Autodesk Inventor part; units mm, degrees
ref_plane "YZ Plane" through (0, 0, 0) normal (1, 0, 0) x (0, 1, 0)
ref_plane "XZ Plane" through (0, 0, 0) normal (0, 1, 0) x (-1, 0, 0)
ref_plane "XY Plane" through (0, 0, 0) normal (0, 0, 1) x (1, 0, 0)
sketch "Sketch1" plane through (0, 0, 0) normal (0, 0, 1) x (1, 0, 0)
  line L0 (-20.32, 1.016) -> (157.7405, 1.016)
  line L1 (-20.32, 1.016) -> (-20.32, 0)
  line L2 (-20.32, 0) -> (174.316, 0)
  line L3 (157.7405, 1.016) -> (158.9661, 1.524)
  line L4 (158.9661, 1.524) -> (174.316, 1.524)
  line L5 (174.316, 1.524) -> (174.316, 0)
  arc A0 (174.316, 1.524) -> (176.856, 4.064) centre (174.316, 4.064) ccw
  line L6 (176.856, 4.064) -> (176.856, 7.009)
  arc A1 (178.38, 7.9375) -> (175.0839, 7.75) centre (177.5921, -7.2764) ccw
  line L7 (176.856, 4.064) -> (179.904, 4.064)
  line L8 (178.38, 4.064) -> (178.38, 7.9375)
  arc A2 (174.316, 0) -> (178.38, 4.064) centre (174.316, 4.064) ccw
  line L9 (175.0839, 7.75) -> (175.0839, 7.3209)
  line L10 (175.0839, 7.3209) -> (176.856, 7.009)
  arc A3 (-19.626, 4.4916) -> (-20.32, 1.016) centre (-11.2701, 1.016) ccw
  line L11 (-19.626, 4.4916) -> (-19.3494, 4.4916)
  line L12 (-19.3494, 4.4916) -> (-18.8257, 3.175)
  line L13 (0, 3.175) -> (4.2213, 3.175)
  line L14 (4.2213, 3.175) -> (5.08, 1.016)
  line L15 (5.08, 1.016) -> (5.08, 0)
  line L16 (0, 3.175) -> (0, 0)
  line L17 (-18.8257, 3.175) -> (0, 3.175)
  line L18 (0, 0) -> (5.08, 0)
  dimension "d1" = 2.032
  dimension "d2" = 3.048
  dimension "d5" = 6.35
  dimension "d11" = 9.0499
  dimension "d12" = 25.4
  dimension "d13" = 5.08
  dimension "d14" = 0.2766
  dimension "d15" = 1.4943
  dimension "d16" = 1.2255
  dimension "d17" = 2.54
  dimension "d18" = 7.9375
  dimension "d19" = 15.2343
  dimension "d20" = 6.5922
  dimension "d21" = 198.7
revolve "Revolution1" add sketch "Sketch1" angle 360 about axis through (-20.32, 0, 0) along (1, 0, 0) contours L15 L2 L16 L0 | L0 L16 L13 L14 | L0 L3 L4 L5 L2 L15 | L16 L2 L1 L0 | L0 A3 L11 L12 L17 L16
sketch "Sketch3" plane through (0, 0, 0) normal (1, 0, 0) x (0, 1, 0)
  circle A0 centre (0, 0) radius 3.175
  line L0 (2.2451, 2.2451) -> (-2.2451, 2.2451)
  line L1 (-2.2451, 2.2451) -> (-2.2451, -2.2451)
  line L2 (-2.2451, -2.2451) -> (2.2451, -2.2451)
  line L3 (2.2451, -2.2451) -> (2.2451, 2.2451)
  point P0 (-0.0045, 0)
extrude "Extrusion1" cut sketch "Sketch3" along normal blind 7.9502 contours A0 L3 | L0 A0 | A0 L2 | L1 A0
revolve "Revolution2" add sketch "Sketch1" angle 360 about axis through (178.38, 4.064, 0) along (0, 1, 0) contours L7 L6 L10 L9 A1 L8
sketch "Sketch2" plane through (174.316, 0, 0) normal (1, 0, 0) x (0, 0, -1)
  circle A0 centre (0, 0) radius 1.524
  line L0 (0, 4.064) -> (3.1623, 4.064)
revolve "Revolution3" add sketch "Sketch2" angle 90 about axis through (174.316, 4.064, 0) along (0, 0, 1)
properties part number "SpokeRear"
Work out the finished part from the listing and answer in its coordinate system (mm). A direction names the side the tool comes from. Round coordinates to 2 decimals unless told otherwise and drop trailing zeros. Write each loop counter-clockwise with the first axis right and the second up, starting at its lowest first coordinate (ties: lowest second). Pieces come first, ordered by that corner, then holes.
1) A cutting plane is placed at A-A (x = 150). Give the vertices of the cut face in (y, z).
2) Straight lines are drawn through the part: line 1 (Z direction, x = 133, y = 0.25); line 2 (X direction, y = -3.75, z = 2). For each, find the intervals that lie inside material, in ascending order.
3) A tool of negligible diameter and unlimited length cuts with its end or side. For faces 1 (the flat face through (2, -2.245, 0)), 2 (the flat face through (2, 0, 2.245)), 3 (the flat face through (2, 2.245, 0)), 4 (the conical face through (157.953, 1.053, 0.332)), from which of +Z, -Z, +X, -X, +Y, -Y can it reach the whole face along a straight path? Write none if from no direction.
4) The mould has two halves that part along X. Classify faces 5 (the cylindrical face through (175.236, 7.532, -0.99)), 6 (the cylindrical face through (166.75, -0.2, 1.51)), 7 (the flat face through (2, 0, -2.245)): pulls with the +X half, pulls with the -X half, needs draft (parallel to the pull), parting line crosses it, or undercut.
5) Given pin 1 Ø2 at (x, z) = (11, -0.5) entering from +Y; pin 2 Ø4 at (x, z) = (18, -0.5) entering from -Y; pin 3 Ø3 at (y, z) = (4.5, -2) entering from -X, each flat-ended and moving along its own axis, determine where each tip first touches the part or whether it passes through.
Completed:
1. outline: circle Ø2.03 at (0, 0)
2. line 1: z = -0.98 to 0.98
2. line 2: x = -19.72 to -19.25
3. face 1: +Z, -Z, +X, -Y
3. face 2: +Z, +X, +Y, -Y
3. face 3: +Z, -Z, +Y
3. face 4: none
4. face 5: parting line crosses it
4. face 6: undercut
4. face 7: needs draft
5. pin 1: stops at y = 1.02
5. pin 2: stops at y = -1.02
5. pin 3: stops at x = -19.99
